Verification items for the finished model (mm, model axes). Face numbers are marked on the shaded views. A direction names the side the tool comes from. Coordinates: 2 decimals unless noted, no trailing zeros. Write each loop counter-clockwise with the first axis right and the second up, starting at its lowest first coordinate (ties: lowest second). Pieces come first, ordered by that corner, then holes. Notation, with made-up numbers: M 81,-36.5 L 131,-36.5 A22 ccw 131,-0.5 Z; hole C 26,6 d11. An arc over 180 degrees is marked long. Answer in a Markdown table with one row per item.
from build123d import *

# Parameters (mm, degrees)
BOSS_EXTRUDE1_DEPTH     = 89
CUT_EXTRUDE1_DEPTH      = 208.523246792
CUT_EXTRUDE1_DEPTH_BACK = 208.523246792
SKETCH3_OUTSIDE_W       = 308.718
SKETCH3_OUTSIDE_H       = 147.718
SHELL1_T                = -3.2


with BuildPart() as part:
    # Sketch2 → Boss-Extrude1 (new body)
    with BuildSketch(Plane.XY):
        with BuildLine():
            Line((-91.428571429, -28.496240602), (-91.428571429, 11.503759398))
            ThreePointArc((-91.428571429, 11.503759398), (-73.8549783, 53.93016627), (-31.428571429, 71.503759398))
            Line((-31.428571429, 71.503759398), (158.571428571, 71.503759398))
            Line((158.571428571, 71.503759398), (158.571428571, -28.496240602))
            Line((158.571428571, -28.496240602), (-91.428571429, -28.496240602))
        make_face()
    extrude(amount=-BOSS_EXTRUDE1_DEPTH)

    # Sketch3 outside → Cut-Extrude1 (cut, two sides: drawn at the far end of the back side and taken through both)
    with BuildSketch(Plane(origin=(0, 71.503759398, 0), x_dir=(1, 0, 0), z_dir=(0, 1, 0)).offset(-CUT_EXTRUDE1_DEPTH_BACK)):
        with Locations((33.571, 44.5)):
            Rectangle(SKETCH3_OUTSIDE_W, SKETCH3_OUTSIDE_H)
        with BuildLine():
            Line((-91.428571429, 0), (98.571428571, 0))
            ThreePointArc((98.571428571, 0), (140.997835443, 17.573593129), (158.571428571, 60))
            Line((158.571428571, 60), (158.571428571, 89))
            Line((158.571428571, 89), (-91.428571429, 89))
            Line((-91.428571429, 89), (-91.428571429, 0))
        make_face(mode=Mode.SUBTRACT)
    extrude(amount=CUT_EXTRUDE1_DEPTH + CUT_EXTRUDE1_DEPTH_BACK, mode=Mode.SUBTRACT)

    # Shell1
    shell1_openings = [part.faces().sort_by_distance(p)[0] for p in [
        (37.130073368, 20.336721461, -89),
    ]]
    offset(amount=SHELL1_T, openings=shell1_openings, kind=Kind.INTERSECTION)


solid = part.part
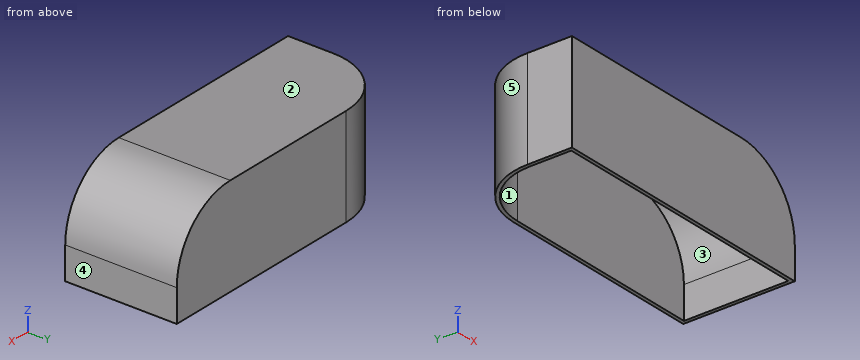
1) Depth check by flat-ended pin: pin 1 (5 mm diameter, centred on y = 56.5, z = -30.5, fed in from -X) (3 decimals); pin 2 (4 mm diameter, centred on x = -40.5, y = -6, fed in from -Z); pin 3 (2 mm diameter, centred on y = -1, z = -42, fed in from +X). Enter the tip coordinate at first touch or a pass-through.
Response values:
| item | result |
|---|---|
| pin 1 | stops at x = -73.785 |
| pin 2 | stops at z = -3.2 |
| pin 3 | stops at x = 156.11 |
2) Tool access check on the marked faces 1 and 2. Record the directions out of +Z, -Z, +X, -X, +Y, -Y that give a thin tool (end or side, any length) a straight path to the whole face; none if there is none.
Response values:
| item | result |
|---|---|
| face 1 | -Z |
| face 2 | +Z, +X, -X, +Y, -Y |
3) Sectioned sample at D-D (z = -36.5). Record the cut outline in (x, y), then the cut area to 3 significant figures.
Response values:
| item | result |
|---|---|
| outline | M -91.43,-28.5 L 153.78,-28.5 L 153.78,71.5 L -31.43,71.5 A60 ccw -91.43,11.5 Z; hole M -88.23,-25.3 L 150.28,-25.3 L 150.28,68.3 L -31.43,68.3 A56.8 ccw -88.23,11.5 Z |
| area | 2,120 mm² |
4) Thickness scan on L1, parallel to Y at x = 7.5, z = -15.5; L2, parallel to Z at x = 33, y = -23.5; L3, parallel to X at y = -7, z = -12.5. Record the ranges inside material, lowest first. Write a range as [from, to].
Response values:
| item | result |
|---|---|
| L1 | y = [-28.5, -25.3], [68.3, 71.5] |
| L2 | z = [-3.2, 0] |
| L3 | x = [-91.43, -88.23], [129.72, 135.23] |
5) Sectioned sample at B-B (x = 44). Record the cut outline in (y, z), then the cut area to 3 significant figures.
Response values:
| item | result |
|---|---|
| outline | M -28.5,-89 L -25.3,-89 L -25.3,-3.2 L 68.3,-3.2 L 68.3,-89 L 71.5,-89 L 71.5,0 L -28.5,0 Z |
| area | 869 mm² |
6) Sectioned sample at A-A (y = -7.5). Record the cut outline in (x, z), then the cut area to 3 significant figures.
Response values:
| item | result |
|---|---|
| outline | M -91.43,-89 L -88.23,-89 L -88.23,-3.2 L 98.57,-3.2 A56.8 cw 155.37,-60 L 155.37,-89 L 158.57,-89 L 158.57,-60 A60 ccw 98.57,0 L -91.43,0 Z |
| area | 1,270 mm² |
7) Sectioned sample at C-C (z = -6). Record the cut outline in (x, y).
Response values:
| item | result |
|---|---|
| outline | M -91.43,-28.5 L 124.72,-28.5 L 124.72,71.5 L -31.43,71.5 A60 ccw -91.43,11.5 Z; hole M -88.23,-25.3 L 116.19,-25.3 L 116.19,68.3 L -31.43,68.3 A56.8 ccw -88.23,11.5 Z |
8) Release check for a two-part mould opening along Y. For the marked faces 3, 4 and 5 record: +Y half, -Y half, draft (parallel to the pull), parting line (faces both ways), or undercut.
Response values:
| item | result |
|---|---|
| face 3 | undercut |
| face 4 | draft |
| face 5 | +Y half |
